Source: CAD feature listing. Evaluate the final solid. Frame: model axes, mm. Give positions to 0.01 mm unless a question says otherwise; leave off trailing zeros. Loops run counter-clockwise (first coordinate to the right, second up) from the corner with the lowest first, then second, coordinate; pieces in that order, holes last.
from build123d import *

# Parameters (mm, degrees)
SKETCH1_W           = 165
SKETCH1_H           = 100
BOSS_EXTRUDE1_DEPTH = 6.35
SKETCH2_R           = 3.175
BOSS_EXTRUDE2_DEPTH = 6.35


with BuildPart() as part:
    # Sketch1 → Boss-Extrude1 (new body)
    with BuildSketch(Plane.XY):
        Rectangle(SKETCH1_W, SKETCH1_H)
    extrude(amount=BOSS_EXTRUDE1_DEPTH)

    # Sketch2 → Boss-Extrude2 (add)
    with BuildSketch(Plane.XY.offset(6.35)):
        with BuildLine():
            Line((-3, 59), (-15, 50))
            Line((-15, 50), (15, 50))
            Line((15, 50), (3, 59))
            ThreePointArc((3, 59), (0, 60), (-3, 59))
        make_face()
        with Locations((0, 55)):
            Circle(SKETCH2_R, mode=Mode.SUBTRACT)
    extrude(amount=-BOSS_EXTRUDE2_DEPTH)


solid = part.part
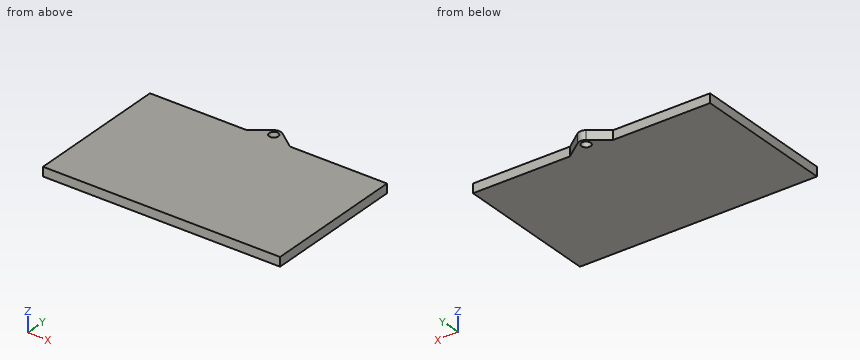
1) Cut plane D-D (x = 60.5). Return loops of the section in (y, z), and give its area (3 significant figures).
Checks:
outline: (-50, 0) - (50, 0) - (50, 6.35) - (-50, 6.35) - close
area: 635 mm2
2) Cut plane C-C (y = 55). Return loops of the section in (x, z) (3 decimals).
Checks:
outline: (-8.333, 0) - (-3.175, 0) - (-3.175, 6.35) - (-8.333, 6.35) - close; (3.175, 0) - (8.333, 0) - (8.333, 6.35) - (3.175, 6.35) - close
3) Contact query for a flat-ended pin moving along its axis: P1, Ø1.9, axis at x = -47, z = 3.5, coming from the +Y side. Output: stop coordinate, or through.
Checks:
P1: stops at y = 50
4) Cut plane B-B (z = 1.5). Return loops of the section in (x, y) (3 decimals).
Checks:
outline: (-82.5, -50) - (82.5, -50) - (82.5, 50) - (15, 50) - (3, 59) arc R5 ccw to (-3, 59) - (-15, 50) - (-82.5, 50) - close; hole circle Ø6.35 at (0, 55)
5) Cut plane A-A (x = 0). Return loops of the section in (y, z) (3 decimals).
Checks:
outline: (-50, 0) - (51.825, 0) - (51.825, 6.35) - (-50, 6.35) - close; (58.175, 0) - (60, 0) - (60, 6.35) - (58.175, 6.35) - close
6) Ray query, probe 1 along Y at (x, z) = (0, 2.75) (3 decimals); probe 2 along Y at (x, z) = (63.5, 2). Return the intervals inside material, ascending.
Checks:
probe 1: y = -50 to 51.825, 58.175 to 60
probe 2: y = -50 to 50
